The listing builds one solid part. Answer for the finished solid, in the listing's coordinates (mm). A direction names the side the tool comes from. Coordinates: 2 decimals unless noted, no trailing zeros. Write each loop counter-clockwise with the first axis right and the second up, starting at its lowest first coordinate (ties: lowest second). Pieces come first, ordered by that corner, then holes.
```python
from build123d import *

# Parameters (mm, degrees)
BOSS_EXTRUDE1_DEPTH = 4
SKETCH3_R           = 4
BOSS_EXTRUDE2_DEPTH = 20
FILLET2_R           = 1


with BuildPart() as part:
    # Sketch2 → Boss-Extrude1 (new body)
    with BuildSketch(Plane.XY):
        Polygon((-10, 0), (-5, -8.660254038), (5, -8.660254038), (10, 0), (5, 8.660254038), (-5, 8.660254038), align=None)
    extrude(amount=BOSS_EXTRUDE1_DEPTH)

    # Sketch3 → Boss-Extrude2 (add)
    with BuildSketch(Plane.XY.offset(4)):
        Circle(SKETCH3_R)
    extrude(amount=BOSS_EXTRUDE2_DEPTH)

    # Fillet2
    fillet2_edges = [part.edges().sort_by_distance(p)[0] for p in [
        (-4, 0, 4),
        (-4, 0, 24),
    ]]
    fillet(fillet2_edges, radius=FILLET2_R)


solid = part.part
```
(1) Section B-B, the plane z = 12.75 is taken. Write down the section's boundary in (x, y), plus the area to 3 significant figures.
(2) Section C-C, the plane y = -7.5 is taken. Write down the section's boundary in (x, z), plus the area to 3 significant figures.
(3) Section A-A, the plane x = 0 is taken. Write down the section's boundary in (y, z), plus the area to 3 significant figures.
(4) Find the intervals of material crossed by probe 1 along Z at (x, y) = (-4.75, -5); probe 2 along Y at (x, z) = (6.5, 1.75); probe 3 along Y at (x, z) = (1, 8.75), in increasing order.
(5) Each of these flat-tipped pins is pushed along its axis until it touches: pin 1 (6 mm diameter, centred on x = -5, y = 4, fed in from +Z); pin 2 (1 mm diameter, centred on y = -5, z = 15.5, fed in from -X); pin 3 (2 mm diameter, centred on y = 1, z = 7, fed in from -X); pin 4 (5 mm diameter, centred on y = -3.5, z = 13, fed in from -X). Where does it stop, or does it pass through?
(6) Which of the six approach directions +Z, -Z, +X, -X, +Y, -Y give full straight-line access (tool end or side, diameter ignored) to faces 1 (the flat face through (4, 4, 4)), 2 (the flat face through (0, 0, 0))?
Solution:
1. outline: circle Ø8 at (0, 0)
1. area: 50.3 mm2
2. outline: (-5.67, 0) - (5.67, 0) - (5.67, 4) - (-5.67, 4) - close
2. area: 45.4 mm2
3. outline: (-8.66, 0) - (8.66, 0) - (8.66, 4) - (5, 4) arc R1 cw to (4, 5) - (4, 23) arc R1 ccw to (3, 24) - (-3, 24) arc R1 ccw to (-4, 23) - (-4, 5) arc R1 cw to (-5, 4) - (-8.66, 4) - close
3. area: 229 mm2
4. probe 1: z = 0 to 4
4. probe 2: y = -6.06 to 6.06
4. probe 3: y = -3.87 to 3.87
5. pin 1: stops at z = 23.92
5. pin 2: passes through
5. pin 3: stops at x = -4
5. pin 4: stops at x = -3.87
6. face 1: +Z
6. face 2: -Z, +X, -X, +Y, -Y
